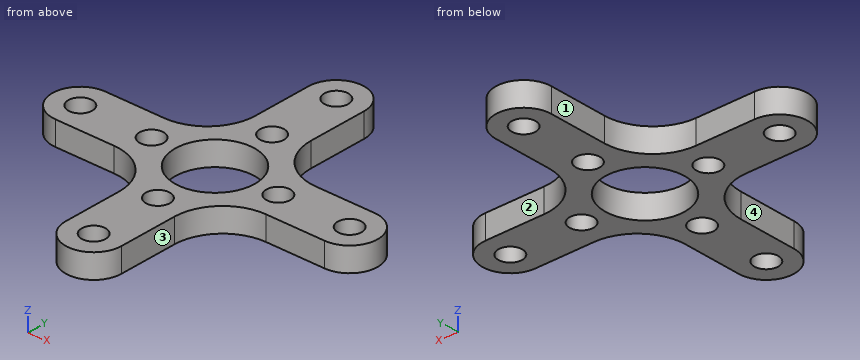
```python
from build123d import *

# Parameters (mm, degrees)
SKETCH1_R           = 5
SKETCH1_R_2         = 1.5
BOSS_EXTRUDE1_DEPTH = 3
CUT_EXTRUDE1_START  = -3
SKETCH2_R           = 1.5
CUT_EXTRUDE1_DEPTH  = 3


with BuildPart() as part:
    # Sketch1 → Boss-Extrude1 (new body)
    with BuildSketch(Plane.XY):
        with BuildLine():
            Line((-3.5, 9.584427843), (-3.5, 17))
            ThreePointArc((-3.5, 17), (0, 20.5), (3.5, 17))
            Line((3.5, 17), (3.5, 9.584427843))
            ThreePointArc((3.5, 9.584427843), (5.282087655, 5.282087655), (9.584427843, 3.5))
            Line((9.584427843, 3.5), (17, 3.5))
            ThreePointArc((17, 3.5), (20.5, 0), (17, -3.5))
            Line((17, -3.5), (9.584427843, -3.5))
            ThreePointArc((9.584427843, -3.5), (5.282087655, -5.282087655), (3.5, -9.584427843))
            Line((3.5, -9.584427843), (3.5, -17))
            ThreePointArc((3.5, -17), (0, -20.5), (-3.5, -17))
            Line((-3.5, -17), (-3.5, -9.584427843))
            ThreePointArc((-3.5, -9.584427843), (-5.282087655, -5.282087655), (-9.584427843, -3.5))
            Line((-9.584427843, -3.5), (-17, -3.5))
            ThreePointArc((-17, -3.5), (-20.5, 0), (-17, 3.5))
            Line((-17, 3.5), (-9.584427843, 3.5))
            ThreePointArc((-9.584427843, 3.5), (-5.282087655, 5.282087655), (-3.5, 9.584427843))
        make_face()
        Circle(SKETCH1_R, mode=Mode.SUBTRACT)
        with Locations((8, 0)):
            Circle(SKETCH1_R_2, mode=Mode.SUBTRACT)
        with Locations((17, 0)):
            Circle(SKETCH1_R_2, mode=Mode.SUBTRACT)
    extrude(amount=BOSS_EXTRUDE1_DEPTH)

    # Sketch2 → Cut-Extrude1 (cut)
    with BuildSketch(Plane.XY.offset(3).offset(CUT_EXTRUDE1_START)):
        with Locations((17, 0)):
            Circle(SKETCH2_R)
        with Locations((8, 0)):
            Circle(SKETCH2_R)
        with Locations((0, -8)):
            Circle(SKETCH2_R)
        with Locations((0, -17)):
            Circle(SKETCH2_R)
        with Locations((-8, 0)):
            Circle(SKETCH2_R)
        with Locations((-17, 0)):
            Circle(SKETCH2_R)
        with Locations((0, 8)):
            Circle(SKETCH2_R)
        with Locations((0, 17)):
            Circle(SKETCH2_R)
    extrude(amount=CUT_EXTRUDE1_DEPTH, mode=Mode.SUBTRACT)


solid = part.part
```
Verification items for the finished model (mm, model axes). Face numbers are marked on the shaded views. A direction names the side the tool comes from. Give positions to 0.01 mm unless a question says otherwise; leave off trailing zeros. Write each loop counter-clockwise with the first axis right and the second up, starting at its lowest first coordinate (ties: lowest second). Pieces come first, ordered by that corner, then holes. Notation, with made-up numbers: M -39.75,5 L -2.75,5 A5 ccw -2.75,10 Z; hole C -0.5,-14 d10. An arc over 180 degrees is marked long. One line per question, with ' | ' between items.
1) Thickness scan on line 1 along X through (y, z) = (-1, 2.8); line 2 along Y through (x, z) = (13, 2.3); line 3 along Y through (x, z) = (-8, 1.8). Record the ranges inside material, lowest first. Write a range as [from, to].
Result:
line 1: x = [-20.35, -18.12], [-15.88, -9.12], [-6.88, -4.9], [4.9, 6.88], [9.12, 15.88], [18.12, 20.35] | line 2: y = [-3.5, 3.5] | line 3: y = [-3.71, -1.5], [1.5, 3.71]
2) Gauge pin test, flat ends, axial feed: pin 1 Ø4 at (x, y) = (-8, 0) entering from -Z; pin 2 Ø0.9 at (y, z) = (14, 1) entering from -X; pin 3 Ø1.5 at (x, z) = (15, 1.5) entering from +Y; pin 4 Ø1.5 at (y, z) = (7.5, 2) entering from +X. Record the tip position at first contact, or that the pin passes through.
Result:
pin 1: stops at z = 0 | pin 2: stops at x = -3.5 | pin 3: stops at y = 3.5 | pin 4: stops at x = 4.2
3) Set-up check for the marked faces 1, 2, 3 and 4: record each of +Z, -Z, +X, -X, +Y, -Y from which the full face is reachable in a straight line by a thin tool's end or side.
Result:
face 1: +Z, -Z, -X, +Y | face 2: +Z, -Z, +X, +Y | face 3: +Z, -Z, +X, -Y | face 4: +Z, -Z, -X, -Y
4) Section check C-C on z = 0.9. State how many separate pieces and enclosed holes the cut face has, plus the area to 3 significant figures.
Result:
separate pieces: 1 | enclosed holes: 9 | area: 401 mm2
5) Section check A-A on y = 0. Enter the section's corners in (x, z), plus the area to 3 significant figures.
Result:
outline: M -20.5,0 L -18.5,0 L -18.5,3 L -20.5,3 Z; M -15.5,0 L -9.5,0 L -9.5,3 L -15.5,3 Z; M -6.5,0 L -5,0 L -5,3 L -6.5,3 Z; M 5,0 L 6.5,0 L 6.5,3 L 5,3 Z; M 9.5,0 L 15.5,0 L 15.5,3 L 9.5,3 Z; M 18.5,0 L 20.5,0 L 20.5,3 L 18.5,3 Z | area: 57.0 mm2
6) Section check D-D on x = 4.5. Enter the section's corners in (y, z), plus the area to 3 significant figures.
Result:
outline: M -6.24,0 L -2.18,0 L -2.18,3 L -6.24,3 Z; M 2.18,0 L 6.24,0 L 6.24,3 L 2.18,3 Z | area: 24.4 mm2
